Source: CAD feature listing. Evaluate the final solid. Frame: model axes, mm. Face numbers are marked on the shaded views. A direction names the side the tool comes from. Round coordinates to 2 decimals unless told otherwise and drop trailing zeros. Write each loop counter-clockwise with the first axis right and the second up, starting at its lowest first coordinate (ties: lowest second). Pieces come first, ordered by that corner, then holes.
from build123d import *

# Parameters (mm, degrees)
SKETCH1_W           = 74.25
SKETCH1_H           = 60
SKETCH1_R           = 3.25
BOSS_EXTRUDE1_DEPTH = 15
SKETCH2_R           = 1.25
CUT_EXTRUDE1_DEPTH  = 82.474305766
CUT_EXTRUDE2_REACH  = 83.474
SKETCH3_R           = 2.5
CUT_EXTRUDE3_DEPTH  = 58.537487806
FILLET1_R           = 10
FILLET2_R           = 0.8


with BuildPart() as part:
    # Sketch1 → Boss-Extrude1 (new body)
    with BuildSketch(Plane(origin=(0, 0, 0), x_dir=(1, 0, 0), z_dir=(0, 1, 0))):
        with Locations((9.625, 0)):
            Rectangle(SKETCH1_W, SKETCH1_H)
        with Locations(Location((36.75, 7.493, 0), (0, 0, 270))):
            Circle(SKETCH1_R, mode=Mode.SUBTRACT)
        with Locations(Location((36.75, -7.493, 0), (0, 0, 270))):
            Circle(SKETCH1_R, mode=Mode.SUBTRACT)
        with BuildLine():
            Line((-1.25, 21.463632032), (-1.25, 25.5))
            Line((-1.25, 25.5), (1.25, 25.5))
            Line((1.25, 25.5), (1.25, 21.463632032))
            ThreePointArc((1.25, 21.463632032), (21.5, 0), (1.25, -21.463632032))
            Line((1.25, -21.463632032), (1.25, -25.5))
            Line((1.25, -25.5), (-1.25, -25.5))
            Line((-1.25, -25.5), (-1.25, -21.463632032))
            ThreePointArc((-1.25, -21.463632032), (-21.5, 0), (-1.25, 21.463632032))
        make_face(mode=Mode.SUBTRACT)
    extrude(amount=BOSS_EXTRUDE1_DEPTH)

    # Sketch2 → Cut-Extrude1 (cut, through all)
    with BuildSketch(Plane.ZY.offset(27.5)):
        with Locations((-23.25, 7.5)):
            Circle(SKETCH2_R)
        with Locations((23.25, 7.5)):
            Circle(SKETCH2_R)
    extrude(amount=-CUT_EXTRUDE1_DEPTH, mode=Mode.SUBTRACT)

    # Cut-Extrude2: up to this face of the body (flat: up to its plane)
    cut_extrude2_end = Plane(part.part.faces().sort_by_distance((-1.25, 7.5, -21.618967883))[0])
    # Sketch3 → Cut-Extrude2 (cut, up to the picked face)
    with BuildSketch(Plane.ZY.offset(27.5), mode=Mode.PRIVATE) as cut_extrude2_sk1:
        with Locations((-23.25, 7.5)):
            Circle(SKETCH3_R)
    cut_extrude2_tool1 = split(extrude(cut_extrude2_sk1.sketch, amount=-CUT_EXTRUDE2_REACH, mode=Mode.PRIVATE), bisect_by=cut_extrude2_end, keep=Keep.BOTH, mode=Mode.PRIVATE)
    # Sketch3 → Cut-Extrude2 (cut, up to the picked face)
    with BuildSketch(Plane.ZY.offset(27.5), mode=Mode.PRIVATE) as cut_extrude2_sk2:
        with Locations((23.25, 7.5)):
            Circle(SKETCH3_R)
    cut_extrude2_tool2 = split(extrude(cut_extrude2_sk2.sketch, amount=-CUT_EXTRUDE2_REACH, mode=Mode.PRIVATE), bisect_by=cut_extrude2_end, keep=Keep.BOTH, mode=Mode.PRIVATE)
    add(cut_extrude2_tool1.solids().sort_by(Axis((-27.5, 7.5, -23.25), (1, 0, 0)))[0], mode=Mode.SUBTRACT)
    add(cut_extrude2_tool2.solids().sort_by(Axis((-27.5, 7.5, 23.25), (1, 0, 0)))[0], mode=Mode.SUBTRACT)

    # Sketch4 → Cut-Extrude3 (cut, through all)
    with BuildSketch(Plane(origin=(0, 15, 0), x_dir=(1, 0, 0), z_dir=(0, 1, 0))):
        Polygon((10.75, -30), (46.75, -14), (46.75, -30), align=None)
    cut_extrude3 = extrude(amount=-CUT_EXTRUDE3_DEPTH, mode=Mode.SUBTRACT)

    # Mirror1: Cut-Extrude3 across plane
    add(cut_extrude3.mirror(Plane.XY), mode=Mode.SUBTRACT)

    # Fillet1
    # the kernel refuses this fillet: 10 mm, written as the material it takes off along each edge
    with BuildSketch(Plane(origin=(46.75, 31.246827227, -14), x_dir=(-0.9138115486202572, 0, -0.4061384660534477), z_dir=(0, -1, 0))) as fillet1_piece_1:
        with BuildLine():
            CenterArc((FILLET1_R * 0.649873089088, -FILLET1_R), FILLET1_R, 90, 66.037511025)
            Line((-FILLET1_R * 0.263938459532, -FILLET1_R * 0.593861533947), (0, 0))
            Line((0, 0), (FILLET1_R * 0.649873089088, 0))
        make_face()
    extrude(amount=47.493654454, mode=Mode.SUBTRACT)
    with BuildSketch(Plane(origin=(10.75, 20.305361261, -30), x_dir=(-1, 0, 0), z_dir=(0, -1, 0)), Plane(origin=(10.75, 20.305361261, 30), x_dir=(0.9138115486202572, 0, -0.4061384660534476), z_dir=(0, -1, 0))) as fillet1_piece_2:
        with BuildLine():
            CenterArc((FILLET1_R * 0.212214450449, -FILLET1_R), FILLET1_R, 90, 23.962488975)
            Line((-FILLET1_R * 0.193924015604, -FILLET1_R * 0.0861884513797), (0, 0))
            Line((0, 0), (FILLET1_R * 0.212214450449, 0))
        make_face()
    extrude(amount=25.610722522, mode=Mode.SUBTRACT)
    with BuildSketch(Plane(origin=(-27.5, -25, 30), x_dir=(0, 0, -1), z_dir=(0, 1, 0)), Plane(origin=(-27.5, -25, -30), x_dir=(1, 0, 0), z_dir=(0, 1, 0))) as fillet1_piece_3:
        with BuildLine():
            CenterArc((FILLET1_R, -FILLET1_R), FILLET1_R, 90, 90)
            Line((0, -FILLET1_R), (0, 0))
            Line((0, 0), (FILLET1_R, 0))
        make_face()
    extrude(amount=65, mode=Mode.SUBTRACT)
    with BuildSketch(Plane(origin=(46.75, 31.246827227, 14), x_dir=(-0.9138115486202572, 0, 0.4061384660534477), z_dir=(0, -1, 0))) as fillet1_piece_4:
        with BuildLine():
            CenterArc((FILLET1_R * 0.649873089088, FILLET1_R), FILLET1_R, 203.962488975, 66.037511025)
            Line((-FILLET1_R * 0.263938459532, FILLET1_R * 0.593861533947), (0, 0))
            Line((0, 0), (FILLET1_R * 0.649873089088, 0))
        make_face()
    extrude(amount=47.493654454, mode=Mode.SUBTRACT)

    # Fillet2
    # the kernel refuses this fillet: 0.8 mm, written as the material it takes off along each edge
    with BuildSketch(Plane(origin=(1.25, -1.854853982, 21.463632032), x_dir=(0.9971801734895888, 0, -0.07504466402932025), z_dir=(0, 1, 0))) as fillet2_piece_1:
        with BuildLine():
            CenterArc((0.742065381, -0.799885177), FILLET2_R, 90.970759103, 84.725452299)
            Line((-0.055678758, -0.739849446), (0, 0))
            ThreePointArc((0, 0), (0.364255838, -0.003085857), (0.728511676, 0))
        make_face()
    extrude(amount=18.709707964, mode=Mode.SUBTRACT)
    with BuildSketch(Plane(origin=(-1.25, -1.854853982, 21.463632032), x_dir=(-0.9971801734895881, 0, -0.07504466402932955), z_dir=(0, 1, 0)), Plane(origin=(-1.25, 7.394114137, 21.463632032), x_dir=(-0.9971801734895881, 0, -0.07504466402932955), z_dir=(0, 1, 0))) as fillet2_piece_2:
        with BuildLine():
            CenterArc((0.742065381, 0.799885177), FILLET2_R, 184.303788597, 84.725452299)
            Line((-0.055678758, 0.739849446), (0, 0))
            ThreePointArc((0, 0), (0.364255838, 0.003085857), (0.728511676, 0))
        make_face()
    extrude(amount=9.460739845, mode=Mode.SUBTRACT)
    with BuildSketch(Plane(origin=(-1.25, 7.394114137, -21.463632032), x_dir=(-0.9971801734895888, 0, 0.07504466402932025), z_dir=(0, 1, 0))) as fillet2_piece_3:
        with BuildLine():
            CenterArc((0.742065381, -0.799885177), FILLET2_R, 90.970759103, 84.725452299)
            Line((-0.055678758, -0.739849446), (0, 0))
            ThreePointArc((0, 0), (0.364255838, -0.003085857), (0.728511676, 0))
        make_face()
    extrude(amount=9.460739845, mode=Mode.SUBTRACT)
    with BuildSketch(Plane(origin=(-1.25, -1.854853982, -21.463632032), x_dir=(0, 0, -1), z_dir=(0, 1, 0))) as fillet2_piece_4:
        with BuildLine():
            CenterArc((0.741941593, 0.8), FILLET2_R, 185.274547701, 84.725452299)
            ThreePointArc((-0.054670914, 0.726457399), (-0.024258302, 0.363460277), (0, 0))
            Line((0, 0), (0.741941593, 0))
        make_face()
    extrude(amount=9.460739845, mode=Mode.SUBTRACT)
    with BuildSketch(Plane(origin=(1.25, -1.854853982, -21.463632032), x_dir=(0, 0, -1), z_dir=(0, 1, 0))) as fillet2_piece_5:
        with BuildLine():
            CenterArc((0.741941593, -0.8), FILLET2_R, 90, 84.725452299)
            ThreePointArc((-0.054670914, -0.726457399), (-0.024258302, -0.363460277), (0, 0))
            Line((0, 0), (0.741941593, 0))
        make_face()
    extrude(amount=18.709707964, mode=Mode.SUBTRACT)


solid = part.part
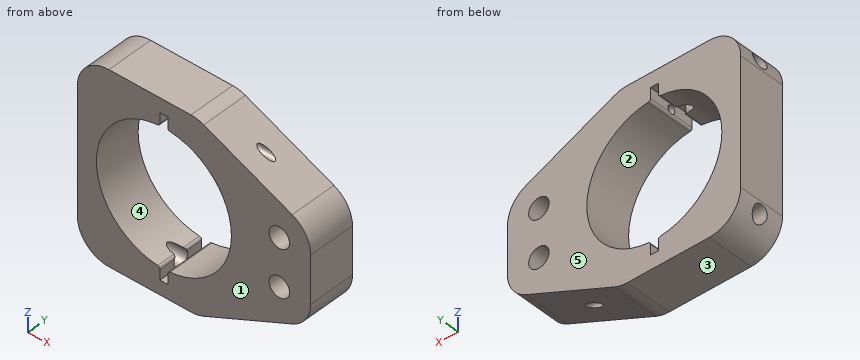
1) Material intervals for line 1 (Y direction, x = -11, z = 23); line 2 (Y direction, x = 11.5, z = 23.25); line 3 (Z direction, x = 34, y = 1.75), sorted ascending.
Taken from the geometry:
line 1: y = 0 to 5.01, 9.99 to 15
line 2: y = 0 to 6.25, 8.75 to 15
line 3: z = -19.67 to -9.23, -5.76 to 5.76, 9.23 to 19.67
2) Section query D-D on z = -23.25. Return the cut outline in (x, y).
Taken from the geometry:
outline: (-26.96, 0) - (-1.25, 0) - (-1.25, 5) - (-26.96, 5) - close; (-26.96, 10) - (-1.25, 10) - (-1.25, 15) - (-26.96, 15) - close; (1.25, 0) - (25.94, 0) - (25.94, 6.25) - (1.25, 6.25) - close; (1.25, 8.75) - (25.94, 8.75) - (25.94, 15) - (1.25, 15) - close
3) Section query B-B on x = -11. Return the cut outline in (y, z).
Taken from the geometry:
outline: (0, -30) - (15, -30) - (15, -18.47) - (0, -18.47) - close; (0, 18.47) - (15, 18.47) - (15, 30) - (0, 30) - close; hole circle Ø5 at (7.5, -23.25); hole circle Ø5 at (7.5, 23.25)
4) Reachability of the marked faces 4 and 5 from +Z, -Z, +X, -X, +Y, -Y: full face, straight path, thin tool, end or side. Return the list, or none.
Taken from the geometry:
face 4: +Y, -Y
face 5: +Z, -Z, +X, -X, +Y
5) Pull-direction query (Z, two-part tool) for the marked faces 1, 2 and 3; classes: released by +Z, released by -Z, zero draft, split by the parting line, or undercut.
Taken from the geometry:
face 1: zero draft
face 2: undercut
face 3: released by -Z
6) Section query C-C on y = 3.75. Return the cut outline in (x, z), then the cut area to 3 significant figures.
Taken from the geometry:
outline: (-27.5, -20) arc R10 ccw to (-17.5, -30) - (8.63, -30) arc R10 ccw to (12.69, -29.14) - (40.81, -16.64) arc R10 ccw to (46.75, -7.5) - (46.75, 7.5) arc R10 ccw to (40.81, 16.64) - (12.69, 29.14) arc R10 ccw to (8.63, 30) - (-17.5, 30) arc R10 ccw to (-27.5, 20) - close; hole (-1.98, -21.41) arc R0.8 cw to (-1.25, -22.21) - (-1.25, -25.5) - (1.25, -25.5) - (1.25, -22.21) arc R0.8 cw to (1.98, -21.41) arc R21.5 ccw to (1.98, 21.41) arc R0.8 cw to (1.25, 22.21) - (1.25, 25.5) - (-1.25, 25.5) - (-1.25, 22.21) arc R0.8 cw to (-1.98, 21.41) arc R21.5 ccw to start; hole circle Ø6.5 at (36.75, -7.49); hole circle Ø6.5 at (36.75, 7.49)
area: 2,280 mm2
7) Section query A-A on z = 2. Return the cut outline in (x, y), then the cut area to 3 significant figures.
Taken from the geometry:
outline: (-27.5, 0) - (-21.41, 0) - (-21.41, 15) - (-27.5, 15) - close; (21.41, 0) - (46.75, 0) - (46.75, 15) - (21.41, 15) - close
area: 472 mm2
8) Contact query for flat-ended pins moving along their axis: P1, Ø1, axis at y = 11, z = -24.5, coming from the +X side; P2, Ø2, axis at y = 7.5, z = -23.25, coming from the +X side; P3, Ø1, axis at y = 11, z = 23.5, coming from the -X side; P4, Ø3, axis at x = 32, y = 11, coming from the -Z side. Output: stop coordinate, or through.
Taken from the geometry:
P1: stops at x = 24.25
P2: passes through
P3: stops at x = -27.04
P4: stops at z = -21.22
